Can you work these out from the model? Positions are in its coordinate system, mm. Give positions to 0.01 mm unless a question says otherwise; leave off trailing zeros. Write each loop counter-clockwise with the first axis right and the second up, starting at its lowest first coordinate (ties: lowest second). Pieces come first, ordered by that corner, then holes.
from build123d import *

# Parameters (mm, degrees)
F1_DEPTH  = 2
F3_DEPTH  = 2.001
F5_D      = 3
F8_DEPTH  = 2
F10_DEPTH = 2
F11_R     = 5
F13_DEPTH = 2.0010001
F14_R     = 3.125
F15_DEPTH = 2.0010001
F17_DEPTH = 2.0010001
F18_R     = 1
F19_R     = 2.5


# Not quite as in the source:
# - a feature names something its author has since deleted; it is built from what else it names


with BuildPart() as f1:
    # F0 (on Top) → F1 (new body)
    with BuildSketch(Plane.XY):
        with BuildLine():
            ThreePointArc((-18.4588585891, 24.3341531066), (-23.2526911935, 23.2526911935), (-24.3341531066, 18.4588585891))
            ThreePointArc((-24.3341531066, 18.4588585891), (-21.9518735553, 9.3657393117), (-21.15, 0))
            ThreePointArc((-21.15, 0), (-21.9518735553, -9.3657393117), (-24.3341531066, -18.4588585891))
            ThreePointArc((-24.3341531066, -18.4588585891), (-23.2526911935, -23.2526911935), (-18.4588585891, -24.3341531066))
            ThreePointArc((-18.4588585891, -24.3341531066), (-9.3657393117, -21.9518735553), (0, -21.15))
            ThreePointArc((0, -21.15), (9.3657393117, -21.9518735553), (18.4588585891, -24.3341531066))
            ThreePointArc((18.4588585891, -24.3341531066), (23.2526911935, -23.2526911935), (24.3341531066, -18.4588585891))
            ThreePointArc((24.3341531066, -18.4588585891), (21.9518735553, -9.3657393117), (21.15, 0))
            ThreePointArc((21.15, 0), (21.9518735553, 9.3657393117), (24.3341531066, 18.4588585891))
            ThreePointArc((24.3341531066, 18.4588585891), (23.2526911935, 23.2526911935), (18.4588585891, 24.3341531066))
            ThreePointArc((18.4588585891, 24.3341531066), (9.3657393117, 21.9518735553), (0, 21.15))
            ThreePointArc((0, 21.15), (-9.3657393117, 21.9518735553), (-18.4588585891, 24.3341531066))
        make_face()
    extrude(amount=F1_DEPTH)

    # F2 (on face) → F3 (cut, through all)
    with BuildSketch(Plane.XY.offset(2)):
        with BuildLine():
            Line((-18.55, -6.5), (-19.35, -6.5))
            ThreePointArc((-19.35, -6.5), (-20.1, -7.25), (-19.35, -8))
            Line((-19.35, -8), (-19.35, -9))
            Line((-19.35, -9), (-19.35, -10))
            ThreePointArc((-19.35, -10), (-20.1, -10.75), (-19.35, -11.5))
            Line((-19.35, -11.5), (-18.55, -11.5))
            Line((-18.55, -11.5), (-17.75, -11.5))
            ThreePointArc((-17.75, -11.5), (-17, -10.75), (-17.75, -10))
            Line((-17.75, -10), (-17.75, -9))
            Line((-17.75, -9), (-17.75, -8))
            ThreePointArc((-17.75, -8), (-17, -7.25), (-17.75, -6.5))
            Line((-17.75, -6.5), (-18.55, -6.5))
        make_face()
        with BuildLine():
            Line((18.55, -11.5), (19.35, -11.5))
            ThreePointArc((19.35, -11.5), (20.1, -10.75), (19.35, -10))
            Line((19.35, -10), (19.35, -9))
            Line((19.35, -9), (19.35, -8))
            ThreePointArc((19.35, -8), (20.1, -7.25), (19.35, -6.5))
            Line((19.35, -6.5), (18.55, -6.5))
            Line((18.55, -6.5), (17.75, -6.5))
            ThreePointArc((17.75, -6.5), (17, -7.25), (17.75, -8))
            Line((17.75, -8), (17.75, -9))
            Line((17.75, -9), (17.75, -10))
            ThreePointArc((17.75, -10), (17, -10.75), (17.75, -11.5))
            Line((17.75, -11.5), (18.55, -11.5))
        make_face()
    extrude(amount=-F3_DEPTH, mode=Mode.SUBTRACT)

    # F5 (through all)
    with Locations(Plane.XY.offset(2)):
        with Locations((-18.3, 8.5), (-20, 20), (20, 20), (18.3, 8.5), (20, -20), (-20, -20)):
            Hole(F5_D / 2)

    # F7 (on Top) → F8 (join, through all)
    with BuildSketch(Plane.XY):
        with BuildLine():
            ThreePointArc((21.0883280757, 24.4694006309), (10.6198106645, 26.3650888705), (0, 27))
            ThreePointArc((0, 27), (-10.6198106645, 26.3650888705), (-21.0883280757, 24.4694006309))
            ThreePointArc((-21.0883280757, 24.4694006309), (-19.7637100249, 24.5939271922), (-18.4588585891, 24.3341531066))
            ThreePointArc((-18.4588585891, 24.3341531066), (-9.3657393117, 21.9518735553), (0, 21.15))
            ThreePointArc((0, 21.15), (9.3657393117, 21.9518735553), (18.4588585891, 24.3341531066))
            ThreePointArc((18.4588585891, 24.3341531066), (19.7637100249, 24.5939271922), (21.0883280757, 24.4694006309))
        make_face()
    extrude(amount=F8_DEPTH)

    # F9 (on Top) → F10 (join, through all)
    with BuildSketch(Plane.XY):
        with BuildLine():
            ThreePointArc((11.6289429392, -26.2381484763), (16.3825233985, -25.4815286377), (21.0883280757, -24.4694006309))
            ThreePointArc((21.0883280757, -24.4694006309), (19.7637100249, -24.5939271922), (18.4588585891, -24.3341531066))
            ThreePointArc((18.4588585891, -24.3341531066), (9.3657393117, -21.9518735553), (0, -21.15))
            ThreePointArc((0, -21.15), (-9.3657393117, -21.9518735553), (-18.4588585891, -24.3341531066))
            ThreePointArc((-18.4588585891, -24.3341531066), (-19.7637100249, -24.5939271922), (-21.0883280757, -24.4694006309))
            ThreePointArc((-21.0883280757, -24.4694006309), (-10.4728212797, -26.3826037941), (0.2960579419, -26.9995083178))
            ThreePointArc((0.2960579419, -26.9995083178), (6.2139125454, -30.3611120266), (11.6289429392, -26.2381484763))
        make_face()
    extrude(amount=F10_DEPTH)

    # F11
    f11_edges = [f1.edges().sort_by_distance(p)[0] for p in [
        (0.296058, -26.999508, 1),
        (11.628943, -26.238148, 1),
    ]]
    fillet(f11_edges, radius=F11_R)

    # F12 (on face) → F13 (cut, through all)
    with BuildSketch(Plane.XY.offset(2)):
        with BuildLine():
            ThreePointArc((11.3, -15.1), (10.55, -14.35), (9.8, -15.1))
            Line((9.8, -15.1), (9.8, -17.4))
            ThreePointArc((9.8, -17.4), (10.55, -18.15), (11.3, -17.4))
            Line((11.3, -17.4), (11.3, -15.1))
        make_face()
        with BuildLine():
            ThreePointArc((1.8, -15.1), (1.05, -14.35), (0.3, -15.1))
            Line((0.3, -15.1), (0.3, -17.4))
            ThreePointArc((0.3, -17.4), (1.05, -18.15), (1.8, -17.4))
            Line((1.8, -17.4), (1.8, -15.1))
        make_face()
        with BuildLine():
            ThreePointArc((15, 19.5), (14.25, 20.25), (13.5, 19.5))
            Line((13.5, 19.5), (13.5, 17.2))
            ThreePointArc((13.5, 17.2), (14.25, 16.45), (15, 17.2))
            Line((15, 17.2), (15, 19.5))
        make_face()
        with BuildLine():
            ThreePointArc((-13.5, 19.5), (-14.25, 20.25), (-15, 19.5))
            Line((-15, 19.5), (-15, 17.2))
            ThreePointArc((-15, 17.2), (-14.25, 16.45), (-13.5, 17.2))
            Line((-13.5, 17.2), (-13.5, 19.5))
        make_face()
    extrude(amount=-F13_DEPTH, mode=Mode.SUBTRACT)

    # F14 (on face) → F15 (cut, through all)
    with BuildSketch(Plane.XY.offset(2)):
        with Locations((5.8, -24.2)):
            Circle(F14_R)
    extrude(amount=-F15_DEPTH, mode=Mode.SUBTRACT)

    # F16 (on face) → F17 (cut, through all)
    with BuildSketch(Plane.XY.offset(2)):
        with BuildLine():
            ThreePointArc((-11.5, 17.2), (-12.3592329599, 15.2031274452), (-14.4, 14.4540939565))
            Line((-14.4, 14.4540939565), (-14.4, -6.5))
            Line((-14.4, -6.5), (0, -6.5))
            Line((0, -6.5), (0, -2))
            Line((0, -2), (14.4, -2))
            Line((14.4, -2), (14.4, 14.4540939565))
            ThreePointArc((14.4, 14.4540939565), (12.3592329599, 15.2031274452), (11.5, 17.2))
            Line((11.5, 17.2), (11.5, 20.2007489844))
            ThreePointArc((11.5, 20.2007489844), (0, 21), (-11.5, 20.2007489844))
            Line((-11.5, 20.2007489844), (-11.5, 17.2))
        make_face()
        with BuildLine():
            ThreePointArc((-14.4, -18.9817306875), (-8.5718756396, -19.8028403577), (-2.7, -20.2057437268))
            Line((-2.7, -20.2057437268), (-2.7, -11.5))
            Line((-2.7, -11.5), (-14.4, -11.5))
            Line((-14.4, -11.5), (-14.4, -18.9817306875))
        make_face()
    extrude(amount=-F17_DEPTH, mode=Mode.SUBTRACT)

    # F18
    f18_edges = [f1.edges().sort_by_distance(p)[0] for p in [
        (-2.7, -11.5, 1),
        (-14.4, -11.5, 1),
        (-14.4, -18.981731, 1),
        (-2.7, -20.205744, 1),
        (11.5, 20.200749, 1),
        (-11.5, 20.200749, 1),
        (-14.4, -6.5, 1),
        (14.4, -2, 1),
        (0, -6.5, 1),
        (-14.4, 14.454094, 1),
        (14.4, 14.454094, 1),
    ]]
    fillet(f18_edges, radius=F18_R)

    # F19
    f19_edges = [f1.edges().sort_by_distance(p)[0] for p in [
        (0, -2, 1),
    ]]
    fillet(f19_edges, radius=F19_R)


solid = f1.part
(1) If I drill on L1, parallel to Y at x = -5, z = 0.2; L2, parallel to X at y = -17, z = 1.95; L3, parallel to Y at x = -20.5, z = 0.2, over which ranges is the centre line in solid material (lowest first)?
Returned:
L1: y = -26.86 to -20.1, -11.5 to -6.5, 20.85 to 26.86
L2: x = -23.84 to -14.4, -2.7 to 0.3, 1.8 to 9.8, 11.3 to 23.84
L3: y = -24.61 to -21.41, -18.59 to 18.59, 21.41 to 24.61
(2) Imagine slicing it at A-A, the plane x = -9.5. Write out the boundary of the cut face in (y, z).
Returned:
outline: (-26.49, 0) - (-19.7, 0) - (-19.7, 2) - (-26.49, 2) - close; (-11.5, 0) - (-6.5, 0) - (-6.5, 2) - (-11.5, 2) - close; (20.46, 0) - (26.49, 0) - (26.49, 2) - (20.46, 2) - close
(3) Will these pins go through, and if not, where does the flat tip stop? P1, Ø1, axis at y = -17, z = 1.5, coming from the +X side; P2, Ø1, axis at x = -4.5, z = 1.5, coming from the -Y side; P3, Ø1.1, axis at y = -5, z = 1, coming from the -X side; P4, Ø1.8, axis at x = 18.3, y = 8.5, coming from the +Z side.
Returned:
P1: stops at x = 24
P2: stops at y = -26.91
P3: stops at x = -21.43
P4: passes through
(4) Imagine slicing it at B-B, the plane y = 5. Write out the boundary of the cut face in (x, z), plus the area to 3 significant figures.
Returned:
outline: (-21.38, 0) - (-14.4, 0) - (-14.4, 2) - (-21.38, 2) - close; (14.4, 0) - (21.38, 0) - (21.38, 2) - (14.4, 2) - close
area: 27.9 mm2
(5) Imagine slicing it at C-C, the plane z = 1.45. Give the number of separate pieces and of enclosed holes in the cut face, plus the area to 3 significant figures.
Returned:
separate pieces: 1
enclosed holes: 15
area: 1,490 mm2
